For this review, take the finished solid that the model builds, in its own axes (mm). Give positions to 0.01 mm unless a question says otherwise; leave off trailing zeros. Write each loop counter-clockwise with the first axis right and the second up, starting at its lowest first coordinate (ties: lowest second). Pieces come first, ordered by that corner, then holes. Notation, with made-up numbers: M 6.25,9.5 L 33.25,9.5 A18 cw 33.25,32.5 Z; hole C 35.5,79 d7. An arc over 180 degrees is marked long. Use one line per item in the form item = value. Start each with the question number.
Q1. Consider section A-A on y = 32. Write out the cut boundary in (x, z).
Q2. Consider section C-C on x = 12. Write out the cut boundary in (y, z), and give its area (3 significant figures).
Q3. Clearance check with flat-ended pins moving along their axes: pin 1 Ø0.6 at (y, z) = (24, 1.5) entering from +X; pin 2 Ø3 at (x, y) = (-11, 7.5) entering from +Z; pin 3 Ø0.6 at (x, z) = (-22, 1) entering from -Y; pin 4 Ø1 at (y, z) = (-23.5, 1.5) entering from -X. State where each tip first meets the part, or that it passes through.
Q4. For probe 1 along X at (y, z) = (26, 0.7); probe 2 along Y at (x, z) = (-32, 1.5); probe 3 along X at (y, z) = (-20.5, 0.8), list the stretches that pass through material, from the lowest coordinate up. Write a range as [from, to].
Q5. Consider section D-D on y = 16. Write out the cut boundary in (x, z), and give its area (3 significant figures).
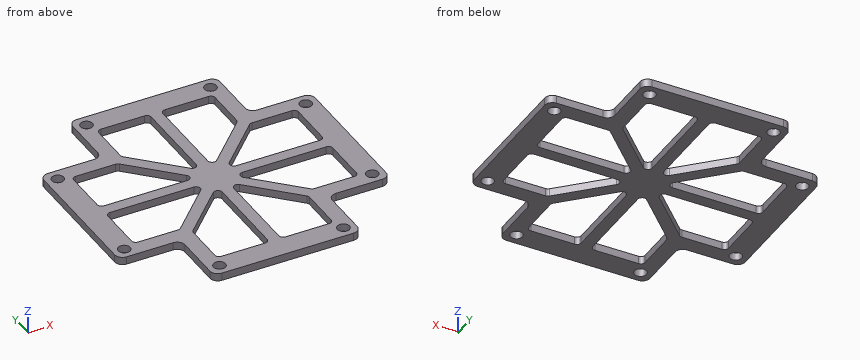
```python
from build123d import *

# Parameters (mm, degrees)
SKETCH_1_W          = 16
SKETCH_1_H          = 38
SKETCH_1_R          = 1.55
SKETCH_1_W_2        = 38
SKETCH_1_H_2        = 16
EXTRUDE_1_DEPTH     = 2
FILLET_1_R          = 2
SKETCH_2_W          = 14
SKETCH_2_H          = 30
SKETCH_2_W_2        = 30
SKETCH_2_H_2        = 14
CUT_EXTRUDE_1_DEPTH = 2
EXTRUDE_2_DEPTH     = 2
FILLET_2_R          = 1.1


with BuildPart() as part:
    # 草图1 → 凸台-拉伸1 (new body)
    # profile 1 of 5: a face of its own
    with BuildSketch(Plane.XY):
        with Locations((-27, 0)):
            Rectangle(SKETCH_1_W, SKETCH_1_H)
        with Locations((-32, -16)):
            Circle(SKETCH_1_R, mode=Mode.SUBTRACT)
        with Locations((-32, 16)):
            Circle(SKETCH_1_R, mode=Mode.SUBTRACT)
    # profile 2 of 5: a face of its own
    with BuildSketch(Plane.XY):
        Rectangle(SKETCH_1_W_2, SKETCH_1_H)
    # profile 3 of 5: a face of its own
    with BuildSketch(Plane.XY):
        with Locations((0, 27)):
            Rectangle(SKETCH_1_W_2, SKETCH_1_H_2)
        with Locations((-16, 32)):
            Circle(SKETCH_1_R, mode=Mode.SUBTRACT)
        with Locations((16, 32)):
            Circle(SKETCH_1_R, mode=Mode.SUBTRACT)
    # profile 4 of 5: a face of its own
    with BuildSketch(Plane.XY):
        with Locations((27, 0)):
            Rectangle(SKETCH_1_W, SKETCH_1_H)
        with Locations((32, -16)):
            Circle(SKETCH_1_R, mode=Mode.SUBTRACT)
        with Locations((32, 16)):
            Circle(SKETCH_1_R, mode=Mode.SUBTRACT)
    # profile 5 of 5: a face of its own
    with BuildSketch(Plane.XY):
        with Locations((0, -27)):
            Rectangle(SKETCH_1_W_2, SKETCH_1_H_2)
        with Locations((-16, -32)):
            Circle(SKETCH_1_R, mode=Mode.SUBTRACT)
        with Locations((16, -32)):
            Circle(SKETCH_1_R, mode=Mode.SUBTRACT)
    extrude(amount=EXTRUDE_1_DEPTH)

    # 圆角1
    fillet_1_edges = [part.edges().sort_by_distance(p)[0] for p in [
        (-19, 19, 1),
        (-19, 35, 1),
        (19, 35, 1),
        (19, 19, 1),
        (35, 19, 1),
        (35, -19, 1),
        (19, -19, 1),
        (19, -35, 1),
        (-19, -35, 1),
        (-19, -19, 1),
        (-35, -19, 1),
        (-35, 19, 1),
    ]]
    fillet(fillet_1_edges, radius=FILLET_1_R)

    # 草图2 → 切除-拉伸1 (cut)
    with BuildSketch(Plane.XY.offset(2)):
        with Locations((-22, 0)):
            Rectangle(SKETCH_2_W, SKETCH_2_H)
        with Locations((22, 0)):
            Rectangle(SKETCH_2_W, SKETCH_2_H)
        Rectangle(SKETCH_2_W_2, SKETCH_2_H)
        with Locations((0, -22)):
            Rectangle(SKETCH_2_W_2, SKETCH_2_H_2)
        with Locations((0, 22)):
            Rectangle(SKETCH_2_W_2, SKETCH_2_H_2)
    extrude(amount=-CUT_EXTRUDE_1_DEPTH, mode=Mode.SUBTRACT)

    # 草图3 → 凸台-拉伸2 (add)
    with BuildSketch(Plane.XY.offset(2)):
        Polygon((-17.121320344, 15), (-3.621320344, 1.5), (-29, 1.5), (-29, -1.5), (-3.621320344, -1.5), (-17.121320344, -15), (-15, -17.121320344), (-1.5, -3.621320344), (-1.5, -29), (1.5, -29), (1.5, -3.621320344), (13.939339828, -16.060660172), (15, -17.121320344), (17.121320344, -15), (16.060660172, -13.939339828), (3.621320344, -1.5), (29, -1.5), (29, 1.5), (3.621320344, 1.5), (17.121320344, 15), (15, 17.121320344), (1.5, 3.621320344), (1.5, 29), (-1.5, 29), (-1.5, 3.621320344), (-15, 17.121320344), align=None)
    extrude(amount=-EXTRUDE_2_DEPTH)

    # 圆角2
    fillet_2_edges = [part.edges().sort_by_distance(p)[0] for p in [
        (-29, -15, 1),
        (-29, 15, 1),
        (-15, 29, 1),
        (15, 29, 1),
        (29, 15, 1),
        (29, -15, 1),
        (15, -29, 1),
        (-15, -29, 1),
        (-17.121320344, 15, 1),
        (-15, 17.121320344, 1),
        (-1.5, 3.621320344, 1),
        (-1.5, 29, 1),
        (1.5, 29, 1),
        (1.5, 3.621320344, 1),
        (15, 17.121320344, 1),
        (17.121320344, 15, 1),
        (3.621320344, 1.5, 1),
        (29, 1.5, 1),
        (29, -1.5, 1),
        (3.621320344, -1.5, 1),
        (17.121320344, -15, 1),
        (15, -17.121320344, 1),
        (1.5, -3.621320344, 1),
        (1.5, -29, 1),
        (-1.5, -29, 1),
        (-1.5, -3.621320344, 1),
        (-15, -17.121320344, 1),
        (-17.121320344, -15, 1),
        (-3.621320344, -1.5, 1),
        (-29, -1.5, 1),
        (-29, 1.5, 1),
        (-3.621320344, 1.5, 1),
    ]]
    fillet(fillet_2_edges, radius=FILLET_2_R)


solid = part.part
```
Working result:
q1.outline = M -19,0 L -17.55,0 L -17.55,2 L -19,2 Z; M -14.45,0 L 14.45,0 L 14.45,2 L -14.45,2 Z; M 17.55,0 L 19,0 L 19,2 L 17.55,2 Z
q2.outline = M -35,0 L -29,0 L -29,2 L -35,2 Z; M -14.12,0 L -9.88,0 L -9.88,2 L -14.12,2 Z; M -1.5,0 L 1.5,0 L 1.5,2 L -1.5,2 Z; M 9.88,0 L 14.12,0 L 14.12,2 L 9.88,2 Z; M 29,0 L 35,0 L 35,2 L 29,2 Z
q2.area = 47.0 mm²
q3.pin_1 = 19
q3.pin_2 = 2
q3.pin_3 = -19
q3.pin_4 = -19
q4.probe_1 = [-19, -15], [-1.5, 1.5], [15, 19]
q4.probe_2 = [-19, -17.55], [-14.45, 14.45], [17.55, 19]
q4.probe_3 = [-19.06, -15], [-1.5, 1.5], [15, 19.06]
q5.outline = M -35,0 L -33.55,0 L -33.55,2 L -35,2 Z; M -30.45,0 L -13.88,0 L -13.88,2 L -30.45,2 Z; M -1.5,0 L 1.5,0 L 1.5,2 L -1.5,2 Z; M 13.88,0 L 30.45,0 L 30.45,2 L 13.88,2 Z; M 33.55,0 L 35,0 L 35,2 L 33.55,2 Z
q5.area = 78.1 mm²
